Source: CAD feature listing. Evaluate the final solid. Frame: model axes, mm. A direction names the side the tool comes from. Give positions to 0.01 mm unless a question says otherwise; leave off trailing zeros. Write each loop counter-clockwise with the first axis right and the second up, starting at its lowest first coordinate (ties: lowest second). Pieces come first, ordered by that corner, then holes. Notation, with made-up numbers: M 3,63.5 L 46,63.5 A23 ccw 46,72.5 Z; hole C 9,4 d4. An arc over 180 degrees is marked long. Answer as a JSON object with one key per item and string values. Group by question number.
```python
from build123d import *

# Parameters (mm, degrees)
SKETCH1_R           = 7.5
BOSS_EXTRUDE1_DEPTH = 18
SKETCH2_W           = 24.164210644
SKETCH2_H           = 2.935838677
CUT_EXTRUDE1_DEPTH  = 3


with BuildPart() as part:
    # Sketch1 → Boss-Extrude1 (new body)
    with BuildSketch(Plane(origin=(0, 0, 0), x_dir=(1, 0, 0), z_dir=(0, 1, 0))):
        Circle(SKETCH1_R)
    extrude(amount=BOSS_EXTRUDE1_DEPTH)

    # Sketch2 → Cut-Extrude1 (cut)
    with BuildSketch(Plane(origin=(0, 18, 0), x_dir=(1, 0, 0), z_dir=(0, 1, 0))):
        with Locations((-0.598960247, 0.431137149)):
            Rectangle(SKETCH2_W, SKETCH2_H)
    extrude(amount=-CUT_EXTRUDE1_DEPTH, mode=Mode.SUBTRACT)


solid = part.part
```
(1) Contact query for flat-ended pins moving along their axis: pin 1 Ø1.5 at (x, y) = (-1.5, 17) entering from -Z; pin 2 Ø3 at (y, z) = (15.5, 5.5) entering from -X; pin 3 Ø2 at (x, y) = (4, 3.5) entering from -Z. Output: stop coordinate, or through.
(2) Section A-A, the plane x = 0. Return loops of the section in (y, z), plus the area to 3 significant figures.
(3) Section B-B, the plane z = 0. Return loops of the section in (x, y).
(4) Section D-D, the plane x = 2.75. Return loops of the section in (y, z).
(5) Access query for faces 1 (the flat face through (0, 0, 0)), 2 (the flat face through (0, 17, -1.899)). Directions: +Z, -Z, +X, -X, +Y, -Y. A direction counts if a zero-diameter tool reaches every point of the face in a straight line with its end or side. Return the directions, or none.
(6) Section C-C, the plane y = 11. Return loops of the section in (x, z).
(7) Ray query, L1, parallel to Z at x = -1, y = 5; L2, parallel to Y at x = 0, z = -1.75; L3, parallel to X at y = 14, z = 6.5. Return the intervals inside material, ascending. Write a range as [from, to].
(8) Pull-direction query (Z, two-part tool) for faces 3 (the flat face through (0, 18, -4)), 4 (the flat face through (0, 17, 1.037)), 5 (the cylindrical face through (6.93, 8.87, 2.87)); classes: pulls with the +Z half, pulls with the -Z half, needs draft (parallel to the pull), parting line crosses it, or undercut.
Reported:
{
 "1": {"pin 1": "stops at z = -7.46", "pin 2": "stops at x = -6.34", "pin 3": "stops at z = -6.87"},
 "2": {"outline": "M 0,-7.5 L 18,-7.5 L 18,-1.9 L 15,-1.9 L 15,1.04 L 18,1.04 L 18,7.5 L 0,7.5 Z", "area": "261 mm2"},
 "3": {"outline": "M -7.5,0 L 7.5,0 L 7.5,15 L -7.5,15 Z"},
 "4": {"outline": "M 0,-6.98 L 18,-6.98 L 18,-1.9 L 15,-1.9 L 15,1.04 L 18,1.04 L 18,6.98 L 0,6.98 Z"},
 "5": {"face 1": "+Z, -Z, +X, -X, -Y", "face 2": "+X, -X, +Y"},
 "6": {"outline": "C 0,0 d15"},
 "7": {"L1": "z = [-7.43, 7.43]", "L2": "y = [0, 15]", "L3": "x = [-3.74, 3.74]"},
 "8": {"face 3": "needs draft", "face 4": "undercut", "face 5": "parting line crosses it"}
}
